Check sheet for the modelled part. Datum: model origin and axes. Units: mm. A direction names the side the tool comes from. Coordinates: 2 decimals unless noted, no trailing zeros. Loops run counter-clockwise (first coordinate to the right, second up) from the corner with the lowest first, then second, coordinate; pieces in that order, holes last. Notation, with made-up numbers: (-5.75, -35.5) -> (24.25, -35.5) arc R24 ccw to (24.25, -9.5) -> close; hole circle Ø3 at (23.5, 76.25). An arc over 180 degrees is marked (long way). Use one line per item in the form item = value.
Autodesk Inventor part; units mm, degrees
ref_plane "YZ Plane" through (0, 0, 0) normal (1, 0, 0) x (0, 1, 0)
ref_plane "XZ Plane" through (0, 0, 0) normal (0, 1, 0) x (-1, 0, 0)
ref_plane "XY Plane" through (0, 0, 0) normal (0, 0, 1) x (1, 0, 0)
sketch "Sketch1" plane through (0, 0, 0) normal (0, 1, 0) x (-1, 0, 0)
  line L0 (20, -4.85) -> (-20, -4.85) construction
  line L1 (-20, -4.85) -> (-20, 4.85) construction
  line L2 (-20, 4.85) -> (20, 4.85) construction
  line L3 (20, 4.85) -> (20, -4.85) construction
  line L4 (0, -4.85) -> (0, 4.85) construction
  line L5 (20, 0) -> (-20, 0) construction
  circle A0 centre (13.5, 0) radius 2.25
  circle A1 centre (-13.5, 0) radius 2.25
  line L6 (67, -18) -> (25, -18) construction
  line L7 (25, -18) -> (25, 18) construction
  line L8 (25, 18) -> (67, 18) construction
  line L9 (67, 18) -> (67, -18) construction
  line L10 (46, -18) -> (46, 18) construction
  line L11 (67, 0) -> (25, 0) construction
  circle A2 centre (61.25, -13) radius 2.75
  circle A3 centre (30.75, -13) radius 2.75
  circle A4 centre (61.25, 13) radius 2.75
  circle A5 centre (30.75, 13) radius 2.75
  line L12 (-67, -18) -> (-25, -18) construction
  line L13 (-25, -18) -> (-25, 18) construction
  line L14 (-25, 18) -> (-67, 18) construction
  line L15 (-67, 18) -> (-67, -18) construction
  line L16 (-46, -18) -> (-46, 18) construction
  line L17 (-67, 0) -> (-25, 0) construction
  circle A6 centre (-61.25, -13) radius 2.75
  circle A7 centre (-30.75, -13) radius 2.75
  circle A8 centre (-61.25, 13) radius 2.75
  circle A9 centre (-30.75, 13) radius 2.75
  line L18 (82, -65) -> (-82, -65)
  line L19 (-82, -65) -> (-82, 65)
  line L20 (-82, 65) -> (82, 65)
  line L21 (82, 65) -> (82, -65)
  point P0 (0, 0)
  point P1 (0, 0)
  dimension "d0" = 40
  dimension "d1" = 9.7
  dimension "d2" = 4.5
  dimension "d3" = 27
  dimension "d4" = 42
  dimension "d6" = 36
  dimension "d7" = 5
  dimension "d8" = 5.5
  dimension "d9" = 30.5
  dimension "d10" = 26
  dimension "d12" = 15
  dimension "d16" = 130
extrude "Extrusion1" add sketch "Sketch1" along normal blind 10
sketch "Sketch5" plane through (-82, 0, -65) normal (-1, 0, 0) x (0, 0, 1)
  line L0 (0, 0) -> (130, 0)
  line L1 (130, 0) -> (130, 10)
  line L2 (0, 10) -> (130, 10)
  line L3 (0, 0) -> (0, 10)
  point P0 (65, 0)
extrude "Extrusion4" add sketch "Sketch5" along normal blind 10
sketch "Sketch6" plane through (0, 10, 0) normal (0, 1, 0) x (1, 0, 0)
  line L0 (-92, 65) -> (-92, -65)
  line L1 (82, -65) -> (-92, -65)
  line L2 (-92, 65) -> (-82, 65)
  line L3 (-82, 65) -> (-82, -65)
  line L4 (-82, -65) -> (-92, -65)
  line L5 (-92, -65) -> (-92, 65)
  point P0 (0, 0)
  dimension "d33" = 10
extrude "Extrusion5" add sketch "Sketch6" along normal blind 80
sketch "Sketch7" plane through (-82, 10, 65) normal (1, 0, 0) x (0, 0, -1)
  line L0 (35, 10) -> (95, 10)
  line L1 (95, 10) -> (95, 70)
  line L2 (95, 70) -> (35, 70)
  line L3 (35, 70) -> (35, 10)
  line L4 (130, 80) -> (0, 80) construction
  line L5 (65, 80) -> (65, 0) construction
  line L6 (62.75, 0) -> (67.25, 0) construction
  line L7 (0, -10) -> (0, 80) construction
  line L8 (130, -10) -> (130, 80) construction
  line L9 (130, 40) -> (0, 40) construction
  point P0 (65, -10)
  dimension "d36" = 60
  dimension "d37" = 60
  dimension "d38" = 40
extrude "Extrusion6" add sketch "Sketch7" along normal blind 10
sketch "Sketch8" plane through (0, 90, 0) normal (0, 1, 0) x (1, 0, 0)
  line L0 (-92, 65) -> (-92, -65)
  line L1 (-92, -65) -> (-82, -65)
  line L2 (-82, -65) -> (-82, 65)
  line L3 (-82, 65) -> (-92, 65)
  point P0 (0, 0)
extrude "Extrusion7" cut sketch "Sketch8" against normal up to surface (10 mm away)
sketch "Sketch9" plane through (-72, 10, 65) normal (1, 0, 0) x (0, 0, -1)
  line L0 (95, 10) -> (95, 70) construction
  line L1 (95, 70) -> (35, 70) construction
  line L2 (35, 70) -> (35, 10) construction
  line L3 (35, 10) -> (95, 10) construction
  line L4 (35, 10) -> (35, 70) construction
  line L5 (35, 40) -> (95, 40) construction
  line L6 (95, 10) -> (95, 70) construction
  line L7 (35, 10) -> (95, 10) construction
  line L8 (65, 10) -> (65, 70) construction
  line L9 (95, 70) -> (35, 70) construction
  line L10 (41.45, 63.55) -> (88.55, 63.55) construction
  line L11 (88.55, 63.55) -> (88.55, 16.45) construction
  line L12 (88.55, 16.45) -> (41.45, 16.45) construction
  line L13 (41.45, 16.45) -> (41.45, 63.55) construction
  circle A0 centre (41.45, 63.55) radius 2.75
  circle A1 centre (41.45, 16.45) radius 2.75
  circle A2 centre (88.55, 16.45) radius 2.75
  circle A3 centre (88.55, 63.55) radius 2.75
  circle A4 centre (65, 40) radius 19.05
  point P0 (65, -10)
  dimension "d43" = 47.1
  dimension "d44" = 47.1
  dimension "d45" = 5.5
  dimension "d46" = 5.5
  dimension "d47" = 5.5
  dimension "d48" = 5.5
  dimension "d51" = 38.1
extrude "Extrusion8" cut sketch "Sketch9" against normal through all
sketch "Sketch10" plane through (-92, 0, -65) normal (-1, 0, 0) x (0, 0, 1)
  circle A0 centre (65, 50) radius 19.05
  line L0 (65, 50) -> (0, 50) construction
  line L1 (0, 10) -> (0, 80)
  line L2 (65, 50) -> (130, 50) construction
  line L3 (130, 10) -> (130, 80)
  line L4 (5, 71.2) -> (33, 71.2) construction
  line L5 (33, 71.2) -> (33, 24.2) construction
  line L6 (33, 24.2) -> (5, 24.2) construction
  line L7 (5, 24.2) -> (5, 71.2) construction
  line L8 (5, 47.7) -> (33, 47.7) construction
  line L9 (65, 50) -> (65, 0) construction
  line L10 (19, 71.2) -> (19, 24.2) construction
  circle A1 centre (19, 65.7) radius 2.75
  circle A2 centre (19, 29.7) radius 2.75
  circle A3 centre (111, 65.7) radius 2.75
  circle A4 centre (111, 29.7) radius 2.75
  point P0 (180, 80)
  dimension "d52" = 28
  dimension "d53" = 47
  dimension "d54" = 2.3
  dimension "d55" = 46
  dimension "d56" = 5.5
  dimension "d57" = 36
extrude "Extrusion9" cut sketch "Sketch10" against normal through all contours A1 | A2 | A3 | A4
sketch "Sketch12" plane through (0, 10, 0) normal (0, 1, 0) x (1, 0, 0)
  line L0 (82, 65) -> (-82, 65)
  line L1 (-82, 65) -> (0, 65)
  line L2 (0, 65) -> (0, 55)
  line L3 (0, 55) -> (-82, 55)
  line L4 (-82, 55) -> (-82, 65)
  line L5 (82, -65) -> (82, 65) construction
  line L6 (82, 0) -> (-92, 0) construction
  line L7 (-92, 65) -> (-92, -65) construction
  line L8 (-82, -65) -> (0, -65)
  line L9 (0, -65) -> (0, -55)
  line L10 (0, -55) -> (-82, -55)
  line L11 (-82, -55) -> (-82, -65)
  point P0 (0, 0)
  dimension "d70" = 82
  dimension "d71" = 10
extrude "Extrusion11" add sketch "Sketch12" along normal up to surface (70 mm away)
chamfer "Chamfer3" distance 70 distance2 82 1 edges at (0, 80, -60) measured on face at (0, 33.3333, -58.3333)
chamfer "Chamfer4" distance 70 distance2 82 1 edges at (0, 80, 60) measured on face at (0, 33.3333, 61.6667)
sketch "Sketch14" plane through (-82, 80, 30) normal (0, 1, 0) x (1, 0, 0)
  line L0 (10, 0) -> (10, 60) construction
  line L1 (-10, 95) -> (-10, -35) construction
  line L2 (10, 0) -> (-10, 0) construction
  line L3 (-10, 0) -> (-10, 60) construction
  line L4 (-10, 60) -> (10, 60) construction
  line L5 (10, 60) -> (10, 0) construction
  line L6 (10, 30) -> (-10, 30) construction
  circle A0 centre (5, 22.5) radius 2.5
  circle A1 centre (5, 37.5) radius 2.5
  point P0 (82, 30)
  dimension "d83" = 60
  dimension "d84" = 5
  dimension "d85" = 15
  dimension "d86" = 15
extrude "Extrusion12" cut sketch "Sketch14" against normal blind 6
sketch "Sketch15" plane through (0, 10, 0) normal (0, 1, 0) x (1, 0, 0)
  line L0 (82, 65) -> (0, 65) construction
  line L1 (82, 65) -> (67, 65) construction
  line L2 (67, 65) -> (67, 50) construction
  line L3 (67, 50) -> (82, 50) construction
  line L4 (82, 50) -> (82, 65) construction
  circle A0 centre (67, 50) radius 2.5
  point P0 (0, 0)
  dimension "d89" = 15
  dimension "d90" = 15
  dimension "d91" = 5
extrude "Extrusion13" cut sketch "Sketch15" against normal blind 6
sketch "Sketch16" plane through (-82, 80, 30) normal (0, 1, 0) x (1, 0, 0)
  line L0 (0, 95) -> (0, 85) construction
  line L1 (-10, 95) -> (-10, -35) construction
  line L2 (0, 85) -> (-10, 85) construction
  line L3 (-10, 85) -> (-10, 80) construction
  line L4 (-10, 80) -> (0, 80) construction
  line L5 (0, 80) -> (0, 85) construction
  circle A0 centre (-5, 80) radius 2.5
  point P0 (82, 30)
  dimension "d94" = 5
  dimension "d95" = 5
extrude "Extrusion14" cut sketch "Sketch16" against normal blind 6
properties part number "positioner_base"
(1) Section check B-B, the plane y = 35.5. Record the boundary of the cut face in (x, z), plus the area to 3 significant figures.
Established:
outline = (-92, -65) -> (-29.87, -65) -> (-29.87, -55) -> (-82, -55) -> (-82, -30) -> (-72, -30) -> (-72, -12.36) -> (-92, -12.36) -> close; (-92, 12.36) -> (-72, 12.36) -> (-72, 30) -> (-82, 30) -> (-82, 55) -> (-29.87, 55) -> (-29.87, 65) -> (-92, 65) -> close
area = 2,450 mm²
(2) Tool access check on faces 1 (the flat face through (-77, 50, -30)), 2 (the flat face through (-4, 0, 1)), 3 (the flat face through (-82, 13, -1)), 4 (the cylindrical face through (-89.5, 77, -50.1)). Record the directions out of +Z, -Z, +X, -X, +Y, -Y that give a thin tool (end or side, any length) a straight path to the whole face; none if there is none.
Established:
face_1 = +X, +Y
face_2 = +Z, -Z, +X, -X, -Y
face_3 = +X
face_4 = +Y
(3) Scan lines: line 1 along Z through (x, y) = (-30.75, 8); line 2 along X through (y, z) = (7.45, -50); line 3 along Z through (x, y) = (67, 7.05). Record each from-to range of solid material in increasing order.
Established:
line_1 = -65 to -15.75, -10.25 to 10.25, 15.75 to 65
line_2 = -92 to 64.5, 69.5 to 82
line_3 = -65 to -52.5, -47.5 to 65
(4) Section check D-D, the plane z = 52. Record the boundary of the cut face in (x, y).
Established:
outline = (-92, 0) -> (82, 0) -> (82, 10) -> (-82, 10) -> (-82, 80) -> (-92, 80) -> close
(5) Section check A-A, the plane x = 30.75. Record the boundary of the cut face in (y, z).
Established:
outline = (0, -65) -> (10, -65) -> (10, -15.75) -> (0, -15.75) -> close; (0, -10.25) -> (10, -10.25) -> (10, 10.25) -> (0, 10.25) -> close; (0, 15.75) -> (10, 15.75) -> (10, 65) -> (0, 65) -> close
(6) Go/stop test with flat-tipped pins: P1, Ø18, axis at y = 57, z = -8, coming from the +X side; P2, Ø4.5, axis at y = 26.45, z = -23.55, coming from the +X side; P3, Ø4, axis at x = 68, z = -49, coming from the +Y side; P4, Ø4, axis at x = -77, z = -7.5, coming from the +Y side. Record where each tip stops, or that it passes through.
Established:
P1 = -72
P2 = through
P3 = 10
P4 = 74
(7) Section check C-C, the plane z = 7.5. Record the boundary of the cut face in (x, y), plus the area to 3 significant figures.
Established:
outline = (-92, 0) -> (82, 0) -> (82, 10) -> (-82, 10) -> (-82, 20) -> (-72, 20) -> (-72, 32.49) -> (-92, 32.49) -> close; (-92, 67.51) -> (-72, 67.51) -> (-72, 80) -> (-74.5, 80) -> (-74.5, 74) -> (-79.5, 74) -> (-79.5, 80) -> (-92, 80) -> close
area = 2,310 mm²
(8) Mould release check, pull along Z, two halves, no side actions. Record for faces 5 (the flat face through (-41.574, 45.49, -59.93)), 6 (the cylindrical face through (64, 5, 13)): +Z half, -Z half, draft (parallel to the pull), parting line (faces both ways), or undercut.
Established:
face_5 = draft
face_6 = undercut
